Geometry check sheet. Reference: drawing and pictorial views, mm from the part's lowest x, y, z. A direction names the side the tool comes from. Give positions to 0.01 mm unless a question says otherwise; leave off trailing zeros. Order: outer loops, then holes, each group sorted by start corner. A loop starts at its lowest first (then second) coordinate and runs counter-clockwise, first axis right, second up. Notation, with made-up numbers: (24, 81) - (82, 81) arc R25 cw to (82, 114) - close; hole circle Ø5 at (41, 46.5). An arc over 180 degrees is marked (long way). Answer as a JSON object with one key per item and string values.
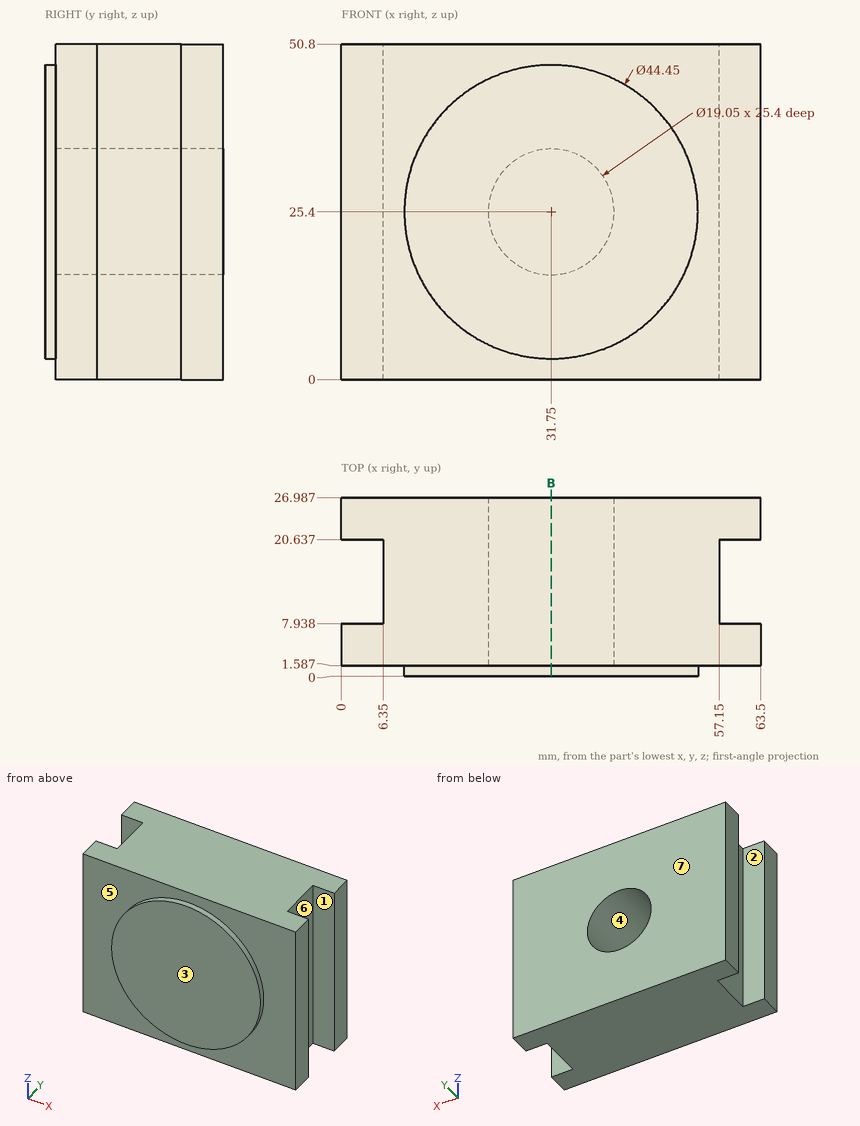
(1) Section check B-B (x = 31.75). Record the cut outline in (y, z) (1 decimal).
Computed values:
{"outline": "(0, 3.2) - (1.6, 3.2) - (1.6, 0) - (27, 0) - (27, 15.9) - (1.6, 15.9) - (1.6, 34.9) - (27, 34.9) - (27, 50.8) - (1.6, 50.8) - (1.6, 47.6) - (0, 47.6) - close"}
(2) Gauge pin test, flat ends, axial feed: pin 1 Ø6.5 at (y, z) = (14.5, 23) entering from -X; pin 2 Ø5 at (y, z) = (14.5, 44.5) entering from +X; pin 3 Ø7 at (x, z) = (61.5, 33) entering from -Y. Record the tip position at first contact, or that the pin passes through.
Computed values:
{"pin 1": "stops at x = 6.35", "pin 2": "stops at x = 57.15", "pin 3": "stops at y = 1.59"}
(3) Release check for a two-part mould opening along Y. For the marked faces 4, 5, 6 and 7 record: pulls with the +Y half, pulls with the -Y half, needs draft (parallel to the pull), parting line crosses it, or undercut.
Computed values:
{"face 4": "needs draft", "face 5": "pulls with the -Y half", "face 6": "undercut", "face 7": "pulls with the +Y half"}
(4) Access from +Z, -Z, +X, -X, +Y, -Y to the whole of each face (thin tool, end or side, straight path). Record for the marked faces 1, 2 and 3.
Computed values:
{"face 1": "+Z, -Z, +X", "face 2": "+Z, -Z, -X", "face 3": "+Z, -Z, +X, -X, -Y"}
(5) Material ranges on line 1 along Z through (x, y) = (31.75, 15.25) (1 decimal); line 2 along Y through (x, z) = (58.5, 9.5); line 3 along Y through (x, z) = (22.5, 27.5), recorded low to high. Write a range as [from, to].
Computed values:
{"line 1": "z = [0, 15.9], [34.9, 50.8]", "line 2": "y = [1.59, 7.94], [20.64, 26.99]", "line 3": "y = [0, 1.59]"}
